from build123d import *

# Parameters (mm, degrees)
EXTRUDE_1_DEPTH     = 2
SKETCH_3_R          = 1.75
CUT_EXTRUDE_1_DEPTH = 10
CHAMFER_1_SIZE      = 3
CHAMFER_2_SIZE      = 1.5


with BuildPart() as part:
    # Эскиз2 → Бобышка-Вытянуть1 (new body)
    with BuildSketch(Plane(origin=(0, 0, 0), x_dir=(1, 0, 0), z_dir=(0, 1, 0))):
        with BuildLine():
            Line((-1.183478947, -7.641318816), (-1.183478947, -30.873613644))
            Line((-1.183478947, -30.873613644), (-21.183478947, -30.873613644))
            Line((-21.183478947, -30.873613644), (-21.183478947, -7.641318816))
            Line((-21.183478947, -7.641318816), (-21.183478947, -7.177217201))
            ThreePointArc((-21.183478947, -7.177217201), (-20.944959731, -5.365483885), (-20.245656774, -3.677217201))
            Line((-20.245656774, -3.677217201), (-16.183478947, 3.358681184))
            Line((-16.183478947, 3.358681184), (-6.183478947, 3.358681184))
            Line((-6.183478947, 3.358681184), (-2.121301121, -3.677217201))
            ThreePointArc((-2.121301121, -3.677217201), (-1.421998163, -5.365483885), (-1.183478947, -7.177217201))
            Line((-1.183478947, -7.177217201), (-1.183478947, -7.641318816))
        make_face()
    extrude(amount=-EXTRUDE_1_DEPTH)

    # Эскиз3 → Вырез-Вытянуть1 (cut)
    with BuildSketch(Plane.XZ.offset(2)):
        with Locations(Location((-11.183478947, 4.141318816, 0), (0, 0, 270))):
            Circle(SKETCH_3_R)
    extrude(amount=-CUT_EXTRUDE_1_DEPTH, mode=Mode.SUBTRACT)

    # Фаска1
    chamfer_1_edges = [part.edges().sort_by_distance(p)[0] for p in [
        (-1.183478947, -1, 30.873613644),
        (-21.183478947, -1, 30.873613644),
    ]]
    chamfer(chamfer_1_edges, length=CHAMFER_1_SIZE)

    # Фаска2
    chamfer_2_edges = [part.edges().sort_by_distance(p)[0] for p in [
        (-11.183478947, -2, 5.891318816),
    ]]
    chamfer(chamfer_2_edges, length=CHAMFER_2_SIZE)


solid = part.part
The listing builds one solid part. Answer for the finished solid, in the listing's coordinates (mm). Give positions to 0.01 mm unless a question says otherwise; leave off trailing zeros. Write each loop counter-clockwise with the first axis right and the second up, starting at its lowest first coordinate (ties: lowest second). Pieces come first, ordered by that corner, then holes.
1) Find the intervals of material crossed by L1, parallel to Y at x = -8.75, z = 4; L2, parallel to X at y = -0.8, z = 6; L3, parallel to Z at x = -10.5, y = -1.7, in increasing order.
2) Section A-A (y = -1.2) is taken. Write down the section's boundary in (x, z), and give its area (3 significant figures).
3) For a pull along X with two mould halves and no side action, classify faces 1 (the face through (-11, -1, 30.874)), 2 (the face through (-1.183, -1, 17)), 3 (the face through (-11.854, -0.254, 2.525)) as pulls with the +X half, pulls with the -X half, needs draft (parallel to the pull), parting line crosses it, or undercut.
4) Section C-C (z = 29) is taken. Write down the section's boundary in (x, y).
5) Section B-B (x = -4.75) is taken. Write down the section's boundary in (y, z).
Response:
1. L1: y = -1.19 to 0
1. L2: x = -21.08 to -12.05, -10.32 to -1.28
1. L3: z = -3.36 to 1.27, 7.01 to 30.87
2. outline: (-21.18, 7.18) arc R7 ccw to (-20.25, 3.68) - (-16.18, -3.36) - (-6.18, -3.36) - (-2.12, 3.68) arc R7 ccw to (-1.18, 7.18) - (-1.18, 27.87) - (-4.18, 30.87) - (-18.18, 30.87) - (-21.18, 27.87) - close; hole circle Ø4.9 at (-11.18, 4.14)
2. area: 613 mm2
3. face 1: needs draft
3. face 2: pulls with the +X half
3. face 3: undercut
4. outline: (-20.06, -2) - (-2.31, -2) - (-2.31, 0) - (-20.06, 0) - close
5. outline: (-2, -0.88) - (0, -0.88) - (0, 30.87) - (-2, 30.87) - close
